Part model, mm, in its own coordinate system. Give positions to 0.01 mm unless a question says otherwise; leave off trailing zeros. Loops run counter-clockwise (first coordinate to the right, second up) from the corner with the lowest first, then second, coordinate; pieces in that order, holes last. Notation, with made-up numbers: (-12, -9) -> (13, -9) arc R34 cw to (13, 28) -> close; hole circle Ø5 at (-23, 38). An arc over 180 degrees is marked (long way). One line per question, with ' | ' between items.
```python
from build123d import *

# Parameters (mm, degrees)
SKETCH1_W           = 28
SKETCH1_H           = 71.2
BOSS_EXTRUDE1_DEPTH = 3
SKETCH4_R           = 1
CUT_EXTRUDE2_DEPTH  = 10
SKETCH5_R           = 4
CUT_EXTRUDE3_DEPTH  = 10
SKETCH7_R           = 1
CUT_EXTRUDE6_DEPTH  = 10
SKETCH8_R           = 1
CUT_EXTRUDE7_DEPTH  = 10
SKETCH10_R          = 1.75
CUT_EXTRUDE9_DEPTH  = 1.6
SKETCH11_R          = 1.75
CUT_EXTRUDE10_DEPTH = 1.6


with BuildPart() as part:
    # Sketch1 → Boss-Extrude1 (new body)
    with BuildSketch(Plane(origin=(0, 0, 0), x_dir=(1, 0, 0), z_dir=(0, 1, 0))):
        Rectangle(SKETCH1_W, SKETCH1_H)
    extrude(amount=BOSS_EXTRUDE1_DEPTH)

    # Sketch4 → Cut-Extrude2 (cut)
    with BuildSketch(Plane(origin=(0, 3, 0), x_dir=(1, 0, 0), z_dir=(0, 1, 0))):
        with Locations((7, -12.8)):
            Circle(SKETCH4_R)
        with Locations((0, -19.8)):
            Circle(SKETCH4_R)
        with Locations((-7, -12.8)):
            Circle(SKETCH4_R)
        with Locations((0, -5.8)):
            Circle(SKETCH4_R)
    extrude(amount=-CUT_EXTRUDE2_DEPTH, mode=Mode.SUBTRACT)

    # Sketch5 → Cut-Extrude3 (cut)
    with BuildSketch(Plane(origin=(0, 3, 0), x_dir=(1, 0, 0), z_dir=(0, 1, 0))):
        with Locations((0, -12.8)):
            Circle(SKETCH5_R)
    extrude(amount=-CUT_EXTRUDE3_DEPTH, mode=Mode.SUBTRACT)

    # Sketch7 → Cut-Extrude6 (cut)
    with BuildSketch(Plane(origin=(0, 3, 0), x_dir=(1, 0, 0), z_dir=(0, 1, 0))):
        with Locations((-9.481224865, -20.948162882)):
            Circle(SKETCH7_R)
        with Locations((-9.248832445, -28.448162882)):
            Circle(SKETCH7_R)
        with Locations((4.518775135, -28.448162882)):
            Circle(SKETCH7_R)
        with Locations((4.518775135, -20.948162882)):
            Circle(SKETCH7_R)
    extrude(amount=-CUT_EXTRUDE6_DEPTH, mode=Mode.SUBTRACT)

    # Sketch8 → Cut-Extrude7 (cut)
    with BuildSketch(Plane(origin=(0, 3, 0), x_dir=(1, 0, 0), z_dir=(0, 1, 0))):
        with Locations((-3.918775135, 28.448162882)):
            Circle(SKETCH8_R)
        with Locations((9.848832445, 28.448162882)):
            Circle(SKETCH8_R)
        with Locations((10.081224865, 20.948162882)):
            Circle(SKETCH8_R)
        with Locations((-3.918775135, 20.948162882)):
            Circle(SKETCH8_R)
    extrude(amount=-CUT_EXTRUDE7_DEPTH, mode=Mode.SUBTRACT)

    # Sketch10 → Cut-Extrude9 (cut)
    with BuildSketch(Plane(origin=(0, 3, 0), x_dir=(1, 0, 0), z_dir=(0, 1, 0))):
        with Locations((0, -19.8)):
            Circle(SKETCH10_R)
        with Locations((-7, -12.8)):
            Circle(SKETCH10_R)
        with Locations((0, -5.8)):
            Circle(SKETCH10_R)
        with Locations((7, -12.8)):
            Circle(SKETCH10_R)
    extrude(amount=-CUT_EXTRUDE9_DEPTH, mode=Mode.SUBTRACT)

    # Sketch11 → Cut-Extrude10 (cut)
    with BuildSketch(Plane.XZ):
        with Locations((-3.918775135, -20.948162882)):
            Circle(SKETCH11_R)
        with Locations((9.848832445, -28.448162882)):
            Circle(SKETCH11_R)
        with Locations((10.081224865, -20.948162882)):
            Circle(SKETCH11_R)
        with Locations((-9.248832445, 28.448162882)):
            Circle(SKETCH11_R)
        with Locations((-9.481224865, 20.948162882)):
            Circle(SKETCH11_R)
        with Locations((4.518775135, 28.448162882)):
            Circle(SKETCH11_R)
        with Locations((4.518775135, 20.948162882)):
            Circle(SKETCH11_R)
        with Locations((-3.918775135, -28.448162882)):
            Circle(SKETCH11_R)
    extrude(amount=-CUT_EXTRUDE10_DEPTH, mode=Mode.SUBTRACT)


solid = part.part
```
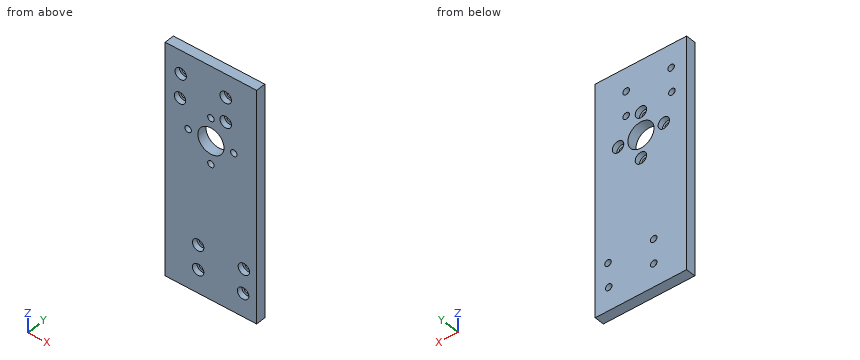
1) Saw through at B-B (z = 12.8). Give the cut face in (x, y).
Found:
outline: (-14, 0) -> (-8, 0) -> (-8, 1.4) -> (-8.75, 1.4) -> (-8.75, 3) -> (-14, 3) -> close; (-6, 0) -> (-4, 0) -> (-4, 3) -> (-5.25, 3) -> (-5.25, 1.4) -> (-6, 1.4) -> close; (4, 0) -> (6, 0) -> (6, 1.4) -> (5.25, 1.4) -> (5.25, 3) -> (4, 3) -> close; (8, 0) -> (14, 0) -> (14, 3) -> (8.75, 3) -> (8.75, 1.4) -> (8, 1.4) -> close
2) Pin check, flat tips, straight feed: P1, Ø1.8, axis at x = -7, z = 12, coming from the +Y side; P2, Ø1.8, axis at x = -9, z = 21.5, coming from the -Y side; P3, Ø1.2, axis at x = 4.52, z = 28.45, coming from the -Y side. Stop position of each tip, or through.
Found:
P1: y = 1.4 | P2: y = 1.6 | P3: through
3) Saw through at C-C (x = 7). Give the cut face in (y, z).
Found:
outline: (0, -35.6) -> (3, -35.6) -> (3, 11.05) -> (1.4, 11.05) -> (1.4, 11.8) -> (0, 11.8) -> close; (0, 13.8) -> (1.4, 13.8) -> (1.4, 14.55) -> (3, 14.55) -> (3, 35.6) -> (0, 35.6) -> close
4) Saw through at D-D (y = 0.7). State how many separate pieces and enclosed holes the cut face has, and give its area (3 significant figures).
Found:
separate pieces: 1 | enclosed holes: 13 | area: 1,850 mm2
5) Drill centre lines: line 1 (X direction, y = 2.15, z = 12.8); line 2 (Z direction, x = 0, y = 1.85); line 3 (X direction, y = 0.6, z = 22.5). Where is each one in solid material? Low to high.
Found:
line 1: -14 to -8.75, -5.25 to -4, 4 to 5.25, 8.75 to 14 | line 2: -35.6 to 4.05, 7.55 to 8.8, 16.8 to 18.05, 21.55 to 35.6 | line 3: -14 to -10.29, -8.67 to 3.71, 5.33 to 14
6) Saw through at A-A (x = 0). Give the cut face in (y, z), and give its area (3 significant figures).
Found:
outline: (0, -35.6) -> (3, -35.6) -> (3, 4.05) -> (1.4, 4.05) -> (1.4, 4.8) -> (0, 4.8) -> close; (0, 6.8) -> (1.4, 6.8) -> (1.4, 7.55) -> (3, 7.55) -> (3, 8.8) -> (0, 8.8) -> close; (0, 16.8) -> (3, 16.8) -> (3, 18.05) -> (1.4, 18.05) -> (1.4, 18.8) -> (0, 18.8) -> close; (0, 20.8) -> (1.4, 20.8) -> (1.4, 21.55) -> (3, 21.55) -> (3, 35.6) -> (0, 35.6) -> close | area: 173 mm2
